```python
from build123d import *

# Parameters (mm, degrees)
EXTRUDE_1_DEPTH = 10
M4X0_71_D       = 3.3
FILLET_2_R      = 2


with BuildPart() as part:
    # Эскиз1 → Бобышка-Вытянуть1 (new body)
    with BuildSketch(Plane.XY):
        with BuildLine():
            Line((-31.75, 0), (-11.05, 0))
            ThreePointArc((-11.05, 0), (-1.514286407, -10.945749708), (10.634965914, -3))
            Line((10.634965914, -3), (31.75, -3))
            Line((31.75, -3), (31.75, -18))
            Line((31.75, -18), (-31.75, -18))
            Line((-31.75, -18), (-31.75, 0))
        make_face()
    extrude(amount=EXTRUDE_1_DEPTH)

    # Отверстие обработанное метчиком M4x0.71 (through all)
    with Locations(Plane(origin=(0, -18, 0), x_dir=(-1, 0, 0), z_dir=(0, -1, 0))):
        with Locations((26.75, -5), (-26.75, -5)):
            Hole(M4X0_71_D / 2)

    # Скругление2
    fillet_2_edges = [part.edges().sort_by_distance(p)[0] for p in [
        (-11.05, 0, 5),
        (10.634965914, -3, 5),
    ]]
    fillet(fillet_2_edges, radius=FILLET_2_R)


solid = part.part
```
Could you check a few things on this model? Use its own coordinates, in mm. A direction names the side the tool comes from. Coordinates: 2 decimals unless noted, no trailing zeros. Write each loop counter-clockwise with the first axis right and the second up, starting at its lowest first coordinate (ties: lowest second). Pieces come first, ordered by that corner, then holes. Notation, with made-up numbers: (44, -19.75) - (90, -19.75) arc R27 cw to (90, 12.25) - close; hole circle Ø6 at (87.5, 19). An arc over 180 degrees is marked (long way). Use a Markdown table: item, result.
Q1. Imagine slicing it at C-C (y = -13.5). List the corners of the cut face in (x, z) for me, and give its area (3 significant figures).
Geometry check:
| item | result |
|---|---|
| outline | (-31.75, 0) - (31.75, 0) - (31.75, 10) - (-31.75, 10) - close; hole circle Ø3.3 at (-26.75, 5); hole circle Ø3.3 at (26.75, 5) |
| area | 618 mm2 |
Q2. Imagine slicing it at D-D (y = -5.25). List the corners of the cut face in (x, z) for me.
Geometry check:
| item | result |
|---|---|
| outline | (-31.75, 0) - (-9.72, 0) - (-9.72, 10) - (-31.75, 10) - close; (9.72, 0) - (31.75, 0) - (31.75, 10) - (9.72, 10) - close; hole circle Ø3.3 at (-26.75, 5); hole circle Ø3.3 at (26.75, 5) |
Q3. Imagine slicing it at B-B (x = 26.75). List the corners of the cut face in (y, z) for me, and give its area (4 significant figures).
Geometry check:
| item | result |
|---|---|
| outline | (-18, 0) - (-3, 0) - (-3, 3.35) - (-18, 3.35) - close; (-18, 6.65) - (-3, 6.65) - (-3, 10) - (-18, 10) - close |
| area | 100.5 mm2 |
Q4. Thinking about a two-plate mould opening in Z: for faces 1 (the flat face through (0, -13, 0)), 2 (the cylindrical face through (-28.4, -8.87, 4.93)), 3 (the cylindrical face through (-1.518, -10.945, 4.93)), which applies, +Z half, -Z half, draft (parallel to the pull), parting line (faces both ways), or undercut?
Geometry check:
| item | result |
|---|---|
| face 1 | -Z half |
| face 2 | undercut |
| face 3 | draft |
Q5. I'm going to push flat-ended pins straight in: pin 1 Ø3 at (x, z) = (26.75, 5) entering from -Y; pin 2 Ø5 at (x, z) = (18.5, 7.5) entering from +Y. Where does each tip first touch, or does it pass through?
Geometry check:
| item | result |
|---|---|
| pin 1 | passes through |
| pin 2 | stops at y = -3 |
Q6. Imagine slicing it at A-A (z = 5). List the corners of the cut face in (x, y) for me.
Geometry check:
| item | result |
|---|---|
| outline | (-31.75, -18) - (-28.4, -18) - (-28.4, 0) - (-31.75, 0) - close; (-25.1, -18) - (25.1, -18) - (25.1, -3) - (12.05, -3) arc R2 ccw to (10.21, -4.23) arc R11.05 cw to (-10.92, -1.69) arc R2 ccw to (-12.9, 0) - (-25.1, 0) - close; (28.4, -18) - (31.75, -18) - (31.75, -3) - (28.4, -3) - close |
Q7. Which directions (+Z, -Z, +X, -X, +Y, -Y) give clear straight access to the entire face, cutting with the end or side of a thin tool? Please do faces 4 (the flat face through (0, -18, 5)), 5 (the cylindrical face through (10.93, -3.346, 5.07)), 6 (the flat face through (22, -3, 5)).
Geometry check:
| item | result |
|---|---|
| face 4 | +Z, -Z, +X, -X, -Y |
| face 5 | +Z, -Z, +Y |
| face 6 | +Z, -Z, +X, +Y |
Q8. Please list where these lines run through material, in increasing order: L1, parallel to X at y = -11.5, z = 5; L2, parallel to Z at x = 26.75, y = -11.75; L3, parallel to X at y = -3.75, z = 5.
Geometry check:
| item | result |
|---|---|
| L1 | x = -31.75 to -28.4, -25.1 to 25.1, 28.4 to 31.75 |
| L2 | z = 0 to 3.35, 6.65 to 10 |
| L3 | x = -31.75 to -28.4, -25.1 to -10.39, 10.49 to 25.1, 28.4 to 31.75 |
